```python
from build123d import *

# Parameters (mm, degrees)
CROQUIS1_R              = 25
SALIENTE_EXTRUIR1_DEPTH = 11.5
CROQUIS2_R              = 16.85
CORTAR_EXTRUIR1_DEPTH   = 2
CROQUIS3_R              = 9.5
CORTAR_EXTRUIR2_DEPTH   = 3.5
CORTAR_EXTRUIR3_REACH   = 37.861
CROQUIS4_R              = 6.5
CROQUIS5_R              = 11
CROQUIS5_R_2            = 6.5
SALIENTE_EXTRUIR2_DEPTH = 1.5
CHAFL_N1_SIZE           = 2


with BuildPart() as part:
    # Croquis1 → Saliente-Extruir1 (new body)
    with BuildSketch(Plane.XY):
        Circle(CROQUIS1_R)
    extrude(amount=-SALIENTE_EXTRUIR1_DEPTH)

    # Croquis2 → Cortar-Extruir1 (cut)
    with BuildSketch(Plane.XY):
        Circle(CROQUIS2_R)
    extrude(amount=-CORTAR_EXTRUIR1_DEPTH, mode=Mode.SUBTRACT)

    # Croquis3 → Cortar-Extruir2 (cut)
    with BuildSketch(Plane.XY.offset(-2)):
        Circle(CROQUIS3_R)
    extrude(amount=-CORTAR_EXTRUIR2_DEPTH, mode=Mode.SUBTRACT)

    # Croquis4 → Cortar-Extruir3 (cut, up to next)
    with BuildSketch(Plane.XY.offset(-5.5), mode=Mode.PRIVATE) as cortar_extruir3_sk1:
        Circle(CROQUIS4_R)
    cortar_extruir3_tool1 = extrude(cortar_extruir3_sk1.sketch, amount=-CORTAR_EXTRUIR3_REACH, mode=Mode.PRIVATE) & part.part
    add(cortar_extruir3_tool1.solids().sort_by_distance((0, 0, -5.5))[0], mode=Mode.SUBTRACT)

    # Croquis5 → Saliente-Extruir2 (add)
    with BuildSketch(Plane(origin=(0, 0, -11.5), x_dir=(-1, 0, 0), z_dir=(0, 0, -1))):
        with Locations(Location((0, 0, 0), (0, 0, 180))):
            Circle(CROQUIS5_R)
        with Locations(Location((0, 0, 0), (0, 0, 180))):
            Circle(CROQUIS5_R_2, mode=Mode.SUBTRACT)
    extrude(amount=SALIENTE_EXTRUIR2_DEPTH)

    # Chaflán1
    chafl_n1_edges = [part.edges().sort_by_distance(p)[0] for p in [
        (-25, 0, 0),
    ]]
    chamfer(chafl_n1_edges, length=CHAFL_N1_SIZE)


solid = part.part
```
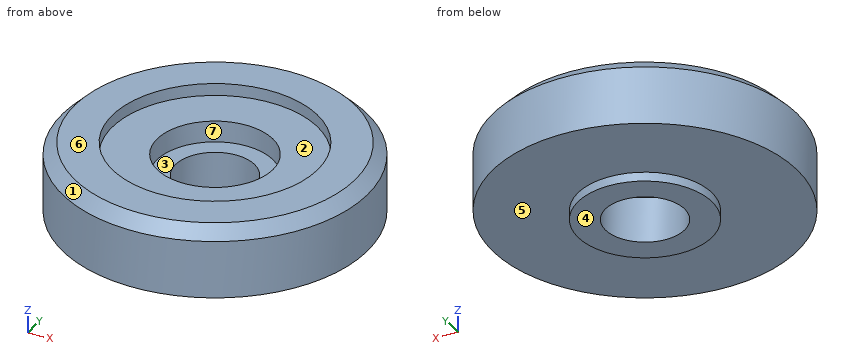
Can you work these out from the model? Positions are in its coordinate system, mm. Face numbers are marked on the shaded views. A direction names the side the tool comes from. Give positions to 0.01 mm unless a question says otherwise; leave off trailing zeros. Loops run counter-clockwise (first coordinate to the right, second up) from the corner with the lowest first, then second, coordinate; pieces in that order, holes last. Notation, with made-up numbers: M 54.25,-32 L 63.25,-32 A12 cw 63.25,-11 Z; hole C 59.25,15.25 d10. An arc over 180 degrees is marked long. Answer in a Markdown table with one row per item.
1. Suppose I cut it at C-C on z = -9.25. Write out the boundary of the cut face in (x, y), plus the area to 3 significant figures.
Taken from the geometry:
| item | result |
|---|---|
| outline | C 0,0 d50; hole C 0,0 d13 |
| area | 1,830 mm² |
2. For pin 1 Ø1.5 at (x, z) = (16, -9) entering from -Y; pin 2 Ø6 at (x, z) = (-8, -3) entering from +Y; pin 3 Ø1.5 at (x, z) = (6.5, -2) entering from +Y, each with a flat end and sliding along its axis, tell me the tip position at first contact or that it passes through.
Taken from the geometry:
| item | result |
|---|---|
| pin 1 | stops at y = -19.81 |
| pin 2 | stops at y = 24.49 |
| pin 3 | stops at y = 24.33 |
3. Suppose I cut it at A-A on x = 0. Write out the boundary of the cut face in (y, z), plus the area to 3 significant figures.
Taken from the geometry:
| item | result |
|---|---|
| outline | M -25,-11.5 L -11,-11.5 L -11,-13 L -6.5,-13 L -6.5,-5.5 L -9.5,-5.5 L -9.5,-2 L -16.85,-2 L -16.85,0 L -23,0 L -25,-2 Z; M 6.5,-13 L 11,-13 L 11,-11.5 L 25,-11.5 L 25,-2 L 23,0 L 16.85,0 L 16.85,-2 L 9.5,-2 L 9.5,-5.5 L 6.5,-5.5 Z |
| area | 373 mm² |
4. If I drill on line 1 along Y through (x, z) = (0, -4.7); line 2 along Y through (x, z) = (0, -9.5); line 3 along Z through (x, y) = (16, 11), over which ranges is the centre line in solid material (lowest first)?
Taken from the geometry:
| item | result |
|---|---|
| line 1 | y = -25 to -9.5, 9.5 to 25 |
| line 2 | y = -25 to -6.5, 6.5 to 25 |
| line 3 | z = -11.5 to 0 |
5. Thinking about a two-plate mould opening in Y: for the marked faces 1, 2, 3 and 4, which applies, released by +Y, released by -Y, zero draft, split by the parting line, or undercut?
Taken from the geometry:
| item | result |
|---|---|
| face 1 | split by the parting line |
| face 2 | undercut |
| face 3 | undercut |
| face 4 | zero draft |
6. Suppose I cut it at D-D on z = -4.75. Write out the boundary of the cut face in (x, y), plus the area to 3 significant figures.
Taken from the geometry:
| item | result |
|---|---|
| outline | C 0,0 d50; hole C 0,0 d19 |
| area | 1,680 mm² |
7. Which directions (+Z, -Z, +X, -X, +Y, -Y) give clear straight access to the entire face, cutting with the end or side of a thin tool? Please do the marked faces 5, 6 and 7.
Taken from the geometry:
| item | result |
|---|---|
| face 5 | -Z |
| face 6 | +Z, +X, -X, +Y, -Y |
| face 7 | +Z |
